```python
from build123d import *

# Parameters (mm, degrees)
SKETCH1_W           = 185.42
SKETCH1_H           = 91.44
SKETCH1_R           = 1.524
BOSS_EXTRUDE1_DEPTH = 1.5875
SKETCH2_W           = 45.72
SKETCH2_H           = 69.85
BOSS_EXTRUDE2_DEPTH = 25.4


with BuildPart() as part:
    # Sketch1 → Boss-Extrude1 (new body)
    with BuildSketch(Plane(origin=(0, 0, 0), x_dir=(1, 0, 0), z_dir=(0, 1, 0))):
        with Locations((-3.360446214, 2.811906005)):
            Rectangle(SKETCH1_W, SKETCH1_H)
        with Locations((-93.530446214, 45.991906005)):
            Circle(SKETCH1_R, mode=Mode.SUBTRACT)
        with Locations((86.809553786, 45.991906005)):
            Circle(SKETCH1_R, mode=Mode.SUBTRACT)
        with Locations((86.809553786, -40.368093995)):
            Circle(SKETCH1_R, mode=Mode.SUBTRACT)
        with Locations((-93.530446214, -40.368093995)):
            Circle(SKETCH1_R, mode=Mode.SUBTRACT)
        with Locations((-3.360446214, 45.991906005)):
            Circle(SKETCH1_R, mode=Mode.SUBTRACT)
        with Locations((-3.360446214, -20.048093995)):
            Circle(SKETCH1_R, mode=Mode.SUBTRACT)
    extrude(amount=BOSS_EXTRUDE1_DEPTH)

    # Sketch2 → Boss-Extrude2 (add)
    with BuildSketch(Plane(origin=(0, 1.5875, 0), x_dir=(1, 0, 0), z_dir=(0, 1, 0))):
        with Locations((-70.702750799, 5.188938255)):
            Rectangle(SKETCH2_W, SKETCH2_H)
    extrude(amount=BOSS_EXTRUDE2_DEPTH)


solid = part.part
```
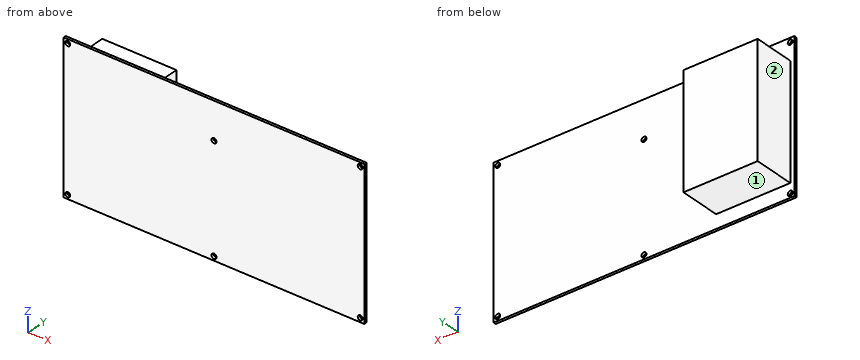
Work out the finished part from the listing and answer in its coordinate system (mm). Face numbers are marked on the shaded views. Give positions to 0.01 mm unless a question says otherwise; leave off trailing zeros. Loops run counter-clockwise (first coordinate to the right, second up) from the corner with the lowest first, then second, coordinate; pieces in that order, holes last. Notation, with made-up numbers: (40.25, 65) -> (49.25, 65) arc R27 ccw to (49.25, 96) -> close; hole circle Ø3 at (-9.5, -25.75). An arc over 180 degrees is marked (long way). Write item = value, one per line. Start each with the question number.
(1) Find section A-A on z = -21.5. Give the vertices of the cut face in (x, y).
(2) Find section B-B on x = -50.5. Give the vertices of the cut face in (y, z), and give its area (3 significant figures).
(3) Find the intervals of material crossed by probe 1 along Y at (x, z) = (41.5, -7.5); probe 2 along X at (y, z) = (17.5, 19); probe 3 along Z at (x, y) = (-50, 24.25), in increasing order. Write a range as from..to.
(4) Find section D-D on x = 9.5. Give the vertices of the cut face in (y, z).
(5) The mould has two halves that part along Z. Classify the marked faces 1 and 2: +Z half, -Z half, draft (parallel to the pull), parting line (faces both ways), or undercut.
(6) Given pin 1 Ø12.5 at (x, y) = (-72, 11) entering from +Z; pin 2 Ø3.5 at (x, z) = (86.81, -45.99) entering from -Y; pin 3 Ø5 at (x, z) = (-3.36, -45.99) entering from +Y; pin 4 Ø5 at (y, z) = (15, -33.5) entering from -X, each flat-ended and moving along its own axis, determine where each tip first touches the part or whether it passes through.
(7) Find section C-C on y = 23.5. Give the vertices of the cut face in (x, z), and give its area (3 significant figures).
From the geometry:
q1.outline = (-96.07, 0) -> (89.35, 0) -> (89.35, 1.59) -> (-47.84, 1.59) -> (-47.84, 26.99) -> (-93.56, 26.99) -> (-93.56, 1.59) -> (-96.07, 1.59) -> close
q2.outline = (0, -48.53) -> (1.59, -48.53) -> (1.59, -40.11) -> (26.99, -40.11) -> (26.99, 29.74) -> (1.59, 29.74) -> (1.59, 42.91) -> (0, 42.91) -> close
q2.area = 1,920 mm^2
q3.probe_1 = 0..1.59
q3.probe_2 = -93.56..-47.84
q3.probe_3 = -40.11..29.74
q4.outline = (0, -48.53) -> (1.59, -48.53) -> (1.59, 42.91) -> (0, 42.91) -> close
q5.face_1 = -Z half
q5.face_2 = draft
q6.pin_1 = 29.74
q6.pin_2 = 0
q6.pin_3 = 1.59
q6.pin_4 = -93.56
q7.outline = (-93.56, -40.11) -> (-47.84, -40.11) -> (-47.84, 29.74) -> (-93.56, 29.74) -> close
q7.area = 3,190 mm^2
